from build123d import *

# Parameters (mm, degrees)
SKETCH_1_W             = 15
SKETCH_1_H             = 15
SKETCH_1_W_2           = 13
SKETCH_1_H_2           = 13
EXTRUDE_1_DEPTH        = 175
SKETCH_2_R             = 1.5
CUT_EXTRUDE_1_DEPTH    = 30
SKETCH_3_R             = 1.5
CUT_EXTRUDE_2_DEPTH    = 5
PATTERN_LINEAR_1_COUNT = 12
PATTERN_LINEAR_1_PITCH = 30


with BuildPart() as part:
    # 草图1 → 凸台-拉伸1 (new, symmetric)
    with BuildSketch(Plane.XY):
        Rectangle(SKETCH_1_W, SKETCH_1_H)
        Rectangle(SKETCH_1_W_2, SKETCH_1_H_2, mode=Mode.SUBTRACT)
    extrude(amount=EXTRUDE_1_DEPTH, both=True)

    # 草图2 → 切除-拉伸1 (cut, symmetric)
    with BuildSketch(Plane.ZY.offset(7.5)):
        with Locations((-160, -2.5)):
            Circle(SKETCH_2_R)
        with Locations((160, -2.5)):
            Circle(SKETCH_2_R)
    extrude(amount=CUT_EXTRUDE_1_DEPTH, both=True, mode=Mode.SUBTRACT)

    # 草图3 → 切除-拉伸2 (cut)
    with BuildSketch(Plane(origin=(0, 7.5, 0), x_dir=(1, 0, 0), z_dir=(0, 1, 0))):
        with Locations(Location((0, -167.5, 0), (0, 0, 270))):
            Circle(SKETCH_3_R)
    cut_extrude_2 = extrude(amount=-CUT_EXTRUDE_2_DEPTH, mode=Mode.SUBTRACT)

    # 阵列(线性)1: 切除-拉伸2 ×12
    with Locations(*[(0, 0, -i * PATTERN_LINEAR_1_PITCH) for i in range(1, PATTERN_LINEAR_1_COUNT)]):
        add(cut_extrude_2, mode=Mode.SUBTRACT)


solid = part.part
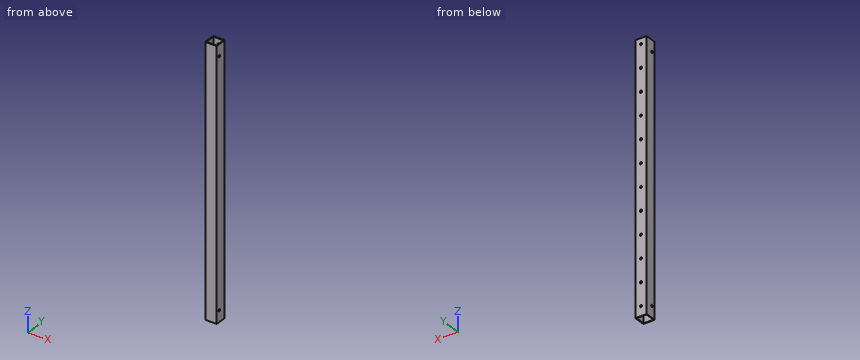
Check sheet for the modelled part. Datum: model origin and axes. Units: mm. Give positions to 0.01 mm unless a question says otherwise; leave off trailing zeros. Order: outer loops, then holes, each group sorted by start corner. A loop starts at its lowest first (then second) coordinate and runs counter-clockwise, first axis right, second up. Notation, with made-up numbers: (38.5, 23.5) - (47.5, 23.5) arc R12 cw to (47.5, 35.5) - close; hole circle Ø4 at (8.25, -11). An arc over 180 degrees is marked (long way). Answer as CSV lines item,"result".
1. Go/stop test with flat-tipped pins: P1, Ø2.5, axis at x = 0, z = 77.5, coming from the +Y side; P2, Ø1.8, axis at y = -2.5, z = 160, coming from the -X side. Record where each tip stops, or that it passes through.
Result sheet:
P1,"y = -6.5"
P2,"through"
2. Scan lines: probe 1 along Y at (x, z) = (-4.5, 59.5); probe 2 along Y at (x, z) = (6.8, -160). Record each from-to range of solid material in increasing order. Write a range as from..to.
Result sheet:
probe 1,"-7.5..-6.5, 6.5..7.5"
probe 2,"-7.5..-4, -1..7.5"
3. Section check A-A (z = 55). Record the boundary of the cut face in (x, y).
Result sheet:
outline,"(-7.5, -7.5) - (7.5, -7.5) - (7.5, 7.5) - (-7.5, 7.5) - close; hole (-6.5, -6.5) - (6.5, -6.5) - (6.5, 6.5) - (-6.5, 6.5) - close"
